Here's how the part is built. I have some questions about the finished solid (model axes, mm). Give positions to 0.01 mm unless a question says otherwise; leave off trailing zeros. Order: outer loops, then holes, each group sorted by start corner. A loop starts at its lowest first (then second) coordinate and runs counter-clockwise, first axis right, second up. Notation, with made-up numbers: M -3,59.25 L 49,59.25 A10 ccw 49,63.25 Z; hole C 69,51.25 d5. An arc over 180 degrees is marked long. One line per item, written item: value. Start each with the question number.
from build123d import *

# Parameters (mm, degrees)
SKETCH001_R  = 3.5
POCKET_DEPTH = 2.2


with BuildPart() as part:
    # Sketch → Revolution (revolve)
    with BuildSketch(Plane.XZ):
        Polygon((1.5, 0), (1.25, 0.144338), (1.25, 2.055662), (1.5, 2.2), (2.65, 2.2), (3.5, 1.709252), (3.5, 0.490748), (2.65, 0), align=None)
    revolve(axis=Axis((0, 0, 0), (0, 0, 1)))

    # Sketch001 → Pocket (cut)
    with BuildSketch(Plane(origin=(0, 0, 2.2), x_dir=(-1, 0, 0), z_dir=(0, 0, 1))):
        Circle(SKETCH001_R)
        Polygon((-2.75, 1.587713), (-2.75, -1.587713), (0, -3.175426), (2.75, -1.587713), (2.75, 1.587713), (0, 3.175426), align=None, mode=Mode.SUBTRACT)
    extrude(amount=-POCKET_DEPTH, mode=Mode.SUBTRACT)


solid = part.part
Item 1: We'd pull the mould along Y, two halves only. Please class faces 1 (the face through (-0.27, -1.22, 1.11)), 2 (the face through (1.36, -2.39, 1.11)), 3 (the face through (-2.75, 0, 1)): +Y half, -Y half, draft (parallel to the pull), parting line (faces both ways), or undercut.
Item 2: Will this pin go through, and if not, where does the flat tip stop? P1, Ø1, axis at x = -1, z = 0.5, coming from the +Y side.
Item 3: I want a section at A-A on y = 0. Write out the boundary of the cut face in (x, z).
Item 4: I want a section at B-B on z = 0.65. Write out the boundary of the cut face in (x, y).
Item 5: Please list where these lines run through material, in increasing order: probe 1 along Y at (x, z) = (-0.2, 0.7); probe 2 along Y at (x, z) = (0.45, 1.5); probe 3 along Y at (x, z) = (1.7, 1.2). Write a range as [from, to].
Answer below:
1. face 1: undercut
1. face 2: -Y half
1. face 3: draft
2. P1: stops at y = 2.89
3. outline: M -2.75,0.06 L -2.65,0 L -1.5,0 L -1.25,0.14 L -1.25,2.06 L -1.5,2.2 L -2.65,2.2 L -2.75,2.14 Z; M 1.25,0.14 L 1.5,0 L 2.65,0 L 2.75,0.06 L 2.75,2.14 L 2.65,2.2 L 1.5,2.2 L 1.25,2.06 Z
4. outline: M -2.75,-1.59 L 0,-3.18 L 2.75,-1.59 L 2.75,1.59 L 0,3.18 L -2.75,1.59 Z; hole C 0,0 d2.5
5. probe 1: y = [-3.06, -1.23], [1.23, 3.06]
5. probe 2: y = [-2.92, -1.17], [1.17, 2.92]
5. probe 3: y = [-2.19, 2.19]
